Source: CAD feature listing. Evaluate the final solid. Frame: model axes, mm. Give positions to 0.01 mm unless a question says otherwise; leave off trailing zeros. Loops run counter-clockwise (first coordinate to the right, second up) from the corner with the lowest first, then second, coordinate; pieces in that order, holes last. Notation, with made-up numbers: (75.5, 71) -> (130.5, 71) arc R24 ccw to (130.5, 100) -> close; hole circle Ø10 at (-1, 19). An arc over 180 degrees is marked (long way). Return JSON: item names as keys, results as strings. Group by question number.
(1) Cut plane A-A on y = -21. Return loops of the section in (x, z), then the cut area to 3 significant figures.
(2) Ray query, line 1 (X direction, y = -7.75, z = 1); line 2 (Z direction, x = -0.5, y = -12.5) (3 decimals); line 3 (X direction, y = -15.75, z = -13). Return the intervals inside material, ascending. Write a range as from..to.
(3) Cut plane C-C on x = -6. Return loops of the section in (y, z), then the cut area to 3 significant figures.
(4) Pin query (flat end, axial travel): pin 1 (2 mm diameter, centred on x = 73, z = 19.5, fed in from +Y); pin 2 (10 mm diameter, centred on y = -4, z = -5, fed in from -X); pin 3 (4 mm diameter, centred on y = -8.5, z = 3.5, fed in from +X); pin 4 (8 mm diameter, centred on x = 93, y = -21, fed in from +Z). Return the tip coordinate at first contact, or that it passes through.
(5) Cut plane B-B on z = -16. Return loops of the section in (x, y), then the cut area to 3 significant figures.
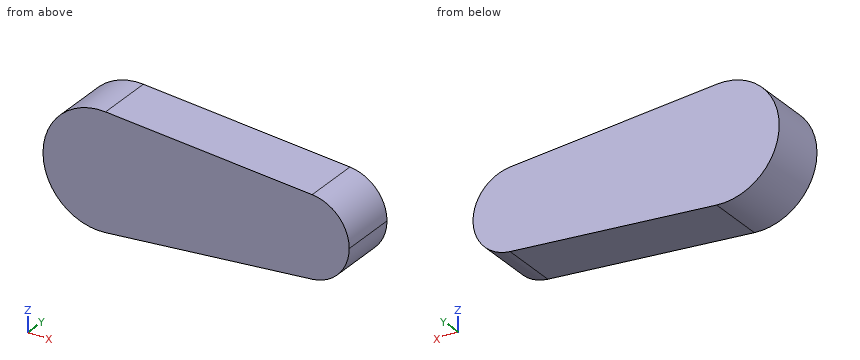
```python
from build123d import *

# Parameters (mm, degrees)
F1_DEPTH = 25


with BuildPart() as f1:
    # F0 (on Front) → F1 (new body)
    with BuildSketch(Plane.XZ):
        with BuildLine():
            ThreePointArc((107.5, 0), (102.879651, 11.847556), (91.458333, 17.43913))
            ThreePointArc((91.458333, 17.43913), (72.5, 0), (91.458333, -17.43913))
            ThreePointArc((91.458333, -17.43913), (102.879651, -11.847556), (107.5, 0))
        make_face()
        with BuildLine():
            ThreePointArc((2.083333, -24.913043), (18.399502, -16.92508), (25, 0))
            ThreePointArc((25, 0), (18.399502, 16.92508), (2.083333, 24.913043))
            ThreePointArc((2.083333, 24.913043), (-25, 0), (2.083333, -24.913043))
        make_face()
        with BuildLine():
            ThreePointArc((2.083333, 24.913043), (18.399502, 16.92508), (25, 0))
            ThreePointArc((25, 0), (18.399502, -16.92508), (2.083333, -24.913043))
            Line((2.083333, -24.913043), (91.458333, -17.43913))
            ThreePointArc((91.458333, -17.43913), (72.5, 0), (91.458333, 17.43913))
            Line((91.458333, 17.43913), (2.083333, 24.913043))
        make_face()
    extrude(amount=F1_DEPTH)


solid = f1.part
```
Answers:
{
 "1": {"outline": "(2.08, -24.91) -> (91.46, -17.44) arc R17.5 ccw to (91.46, 17.44) -> (2.08, 24.91) arc R25 ccw (long way) to start", "area": "5,300 mm²"},
 "2": {"line 1": "-24.98..107.47", "line 2": "-24.995..24.995", "line 3": "-21.35..101.72"},
 "3": {"outline": "(-25, -24.27) -> (0, -24.27) -> (0, 24.27) -> (-25, 24.27) -> close", "area": "1,210 mm²"},
 "4": {"pin 1": "y = 0", "pin 2": "x = -25", "pin 3": "x = 107.44", "pin 4": "z = 17.64"},
 "5": {"outline": "(-19.21, -25) -> (97.09, -25) -> (97.09, 0) -> (-19.21, 0) -> close", "area": "2,910 mm²"}
}
